from build123d import *

# Parameters (mm, degrees)
BOSS_EXTRUDE1_DEPTH = 50
SKETCH1_3_W         = 42
SKETCH1_3_H         = 21
BOSS_EXTRUDE2_DEPTH = 2
BOSS_EXTRUDE3_START = 50
SKETCH1_4_W         = 42
SKETCH1_4_H         = 21
BOSS_EXTRUDE3_DEPTH = 2
SKETCH2_R           = 4.458076667
CUT_EXTRUDE1_DEPTH  = 2
CHAMFER1_SIZE       = 1
FILLET1_R           = 1


with BuildPart() as part:
    # Sketch1 → Boss-Extrude1 (new body)
    with BuildSketch(Plane.XY):
        Polygon((40, 21), (40, 2), (2, 2), (2, 21), (0, 21), (0, 0), (42, 0), (42, 21), align=None)
    extrude(amount=BOSS_EXTRUDE1_DEPTH)

    # Sketch1<3> → Boss-Extrude2 (add)
    with BuildSketch(Plane.XY):
        with Locations((21, 10.5)):
            Rectangle(SKETCH1_3_W, SKETCH1_3_H)
    extrude(amount=-BOSS_EXTRUDE2_DEPTH)

    # Sketch1<4> → Boss-Extrude3 (add)
    with BuildSketch(Plane.XY.offset(BOSS_EXTRUDE3_START)):
        with Locations((21, 10.5)):
            Rectangle(SKETCH1_4_W, SKETCH1_4_H)
    extrude(amount=BOSS_EXTRUDE3_DEPTH)

    # Sketch2 → Cut-Extrude1 (cut)
    with BuildSketch(Plane(origin=(0, 0, -2), x_dir=(-1, 0, 0), z_dir=(0, 0, -1))):
        with Locations((-21, 10.5)):
            Circle(SKETCH2_R)
    extrude(amount=-CUT_EXTRUDE1_DEPTH, mode=Mode.SUBTRACT)

    # Chamfer1
    chamfer1_edges = [part.edges().sort_by_distance(p)[0] for p in [
        (42, 0, 25),
        (0, 0, 25),
        (42, 10.5, -2),
        (21, 0, -2),
        (0, 10.5, -2),
        (42, 10.5, 52),
        (21, 0, 52),
        (0, 10.5, 52),
    ]]
    chamfer(chamfer1_edges, length=CHAMFER1_SIZE)

    # Fillet1
    # the kernel refuses this fillet: 1 mm, written as the material it takes off along each edge
    with BuildSketch(Plane(origin=(43.5, 21, 52), x_dir=(0, 0, -1), z_dir=(-1, 0, 0))) as fillet1_piece_1:
        with BuildLine():
            CenterArc((FILLET1_R, FILLET1_R), FILLET1_R, 180, 90)
            Line((0, FILLET1_R), (0, 0))
            Line((0, 0), (FILLET1_R, 0))
        make_face()
    extrude(amount=45, mode=Mode.SUBTRACT)
    with BuildSketch(Plane(origin=(0, 21, -3.5), x_dir=(1, 0, 0), z_dir=(0, 0, 1)), Plane(origin=(42, 21, 53.5), x_dir=(-1, 0, 0), z_dir=(0, 0, -1))) as fillet1_piece_2:
        with BuildLine():
            CenterArc((FILLET1_R, -FILLET1_R), FILLET1_R, 90, 90)
            Line((0, -FILLET1_R), (0, 0))
            Line((0, 0), (FILLET1_R, 0))
        make_face()
    extrude(amount=57, mode=Mode.SUBTRACT)
    with BuildSketch(Plane(origin=(43.5, 21, -2), x_dir=(0, 0, 1), z_dir=(-1, 0, 0))) as fillet1_piece_3:
        with BuildLine():
            CenterArc((FILLET1_R, -FILLET1_R), FILLET1_R, 90, 90)
            Line((0, -FILLET1_R), (0, 0))
            Line((0, 0), (FILLET1_R, 0))
        make_face()
    extrude(amount=45, mode=Mode.SUBTRACT)
    with BuildSketch(Plane(origin=(-1.767766953, 21, 0.767766953), x_dir=(0.7071067811865476, 0, 0.7071067811865476), z_dir=(0.7071067811865476, 0, -0.7071067811865476))) as fillet1_piece_4:
        with BuildLine():
            CenterArc((FILLET1_R, FILLET1_R), FILLET1_R, 180, 90)
            Line((0, FILLET1_R), (0, 0))
            Line((0, 0), (FILLET1_R, 0))
        make_face()
    extrude(amount=6.414213562, mode=Mode.SUBTRACT)
    with BuildSketch(Plane(origin=(43.767766953, 21, 0.767766953), x_dir=(-0.7071067811865475, 0, 0.7071067811865476), z_dir=(-0.7071067811865476, 0, -0.7071067811865476))) as fillet1_piece_5:
        with BuildLine():
            CenterArc((FILLET1_R, -FILLET1_R), FILLET1_R, 90, 90)
            Line((0, -FILLET1_R), (0, 0))
            Line((0, 0), (FILLET1_R, 0))
        make_face()
    extrude(amount=6.414213562, mode=Mode.SUBTRACT)


solid = part.part
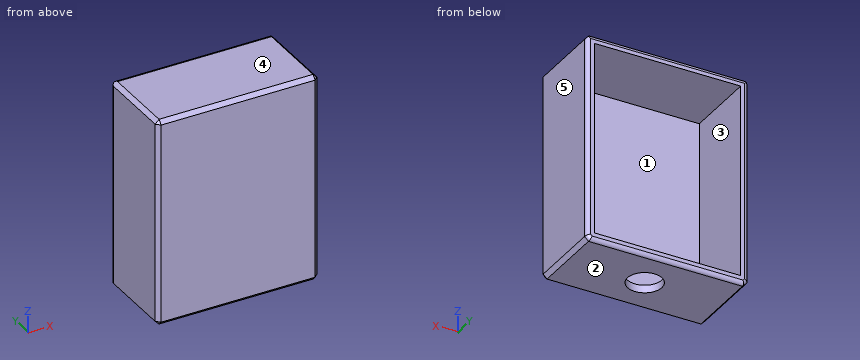
Geometry: final body of the model. Coordinates: model frame, mm. Face numbers are marked on the shaded views. A direction names the side the tool comes from. Give positions to 0.01 mm unless a question says otherwise; leave off trailing zeros. Loops run counter-clockwise (first coordinate to the right, second up) from the corner with the lowest first, then second, coordinate; pieces in that order, holes last. Notation, with made-up numbers: (-33, -22.75) - (-13, -22.75) arc R12 cw to (-13, -13.75) - close; hole circle Ø6 at (2.5, 84.5). An arc over 180 degrees is marked (long way). Answer as CSV lines item,"result". Start each with the question number.
1. Section C-C, the plane z = 16. Return loops of the section in (x, y).
2. Section D-D, the plane x = 12.5. Return loops of the section in (y, z), plus the area to 3 significant figures.
3. Pin query (flat end, axial travel): P1, Ø8, axis at x = 21, y = 10.5, coming from the -Z side; P2, Ø19, axis at x = 16.5, z = 23, coming from the +Y side. Return the tip coordinate at first contact, or that it passes through.
4. Section B-B, the plane y = 5. Return loops of the section in (x, z).
5. Draft query along X for the marked faces 3, 4 and 5. Return one class per face: released by +X, released by -X, zero draft, split by the parting line, or undercut.
6. Reachability of the marked faces 1 and 2 from +Z, -Z, +X, -X, +Y, -Y: full face, straight path, thin tool, end or side. Return the list, or none.
7. Section A-A, the plane x = 21. Return loops of the section in (y, z), plus the area to 3 significant figures.
8. Ray query, L1, parallel to X at y = 17.25, z = 33; L2, parallel to Z at x = 25, y = 20; L3, parallel to Y at x = 21, z = -0.45. Return the intervals inside material, ascending.
Answers:
1,outline,"(0, 1) - (1, 0) - (41, 0) - (42, 1) - (42, 20) arc R1 ccw to (41, 21) - (40, 21) - (40, 2) - (2, 2) - (2, 21) - (1, 21) arc R1 ccw to (0, 20) - close"
2,outline,"(0, -1) - (1, -2) - (20, -2) arc R1 ccw to (21, -1) - (21, 0) - (2, 0) - (2, 50) - (21, 50) - (21, 51) arc R1 ccw to (20, 52) - (1, 52) - (0, 51) - close"
2,area,"183 mm2"
3,P1,"stops at z = 50"
3,P2,"stops at y = 2"
4,outline,"(0, -1) - (1, -2) - (41, -2) - (42, -1) - (42, 51) - (41, 52) - (1, 52) - (0, 51) - close; hole (2, 0) - (40, 0) - (40, 50) - (2, 50) - close"
5,face 3,"undercut"
5,face 4,"zero draft"
5,face 5,"released by +X"
6,face 1,"+Y"
6,face 2,"-Z, +X, -X, +Y, -Y"
7,outline,"(0, -1) - (1, -2) - (6.04, -2) - (6.04, 0) - (2, 0) - (2, 50) - (21, 50) - (21, 51) arc R1 ccw to (20, 52) - (1, 52) - (0, 51) - close; (14.96, -2) - (20, -2) arc R1 ccw to (21, -1) - (21, 0) - (14.96, 0) - close"
7,area,"165 mm2"
8,L1,"x = 0 to 2, 40 to 42"
8,L2,"z = -2 to 0, 50 to 52"
8,L3,"y = 0 to 6.04, 14.96 to 21"
